Source: CAD feature listing. Evaluate the final solid. Frame: model axes, mm. Face numbers are marked on the shaded views. A direction names the side the tool comes from. Give positions to 0.01 mm unless a question says otherwise; leave off trailing zeros. Order: outer loops, then holes, each group sorted by start corner. A loop starts at its lowest first (then second) coordinate and runs counter-clockwise, first axis right, second up. Notation, with made-up numbers: (-38, -22) -> (17, -22) arc R23 cw to (17, 5) -> close; hole circle Ø6 at (34, 24). An arc over 180 degrees is marked (long way). Use CSV: the item, a comma, the result in double quotes.
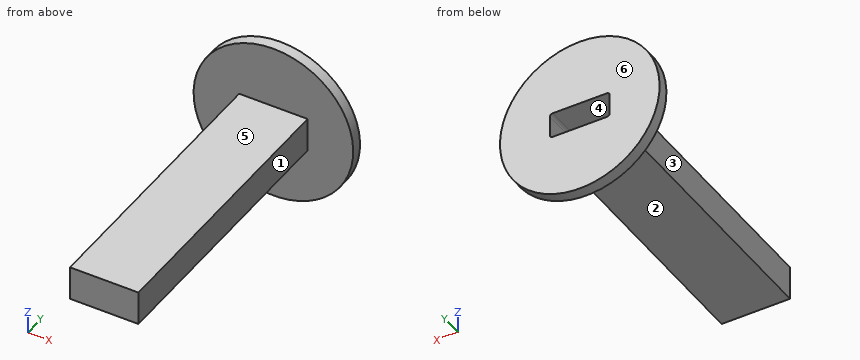
```python
from build123d import *

# Parameters (mm, degrees)
SKETCH1_R           = 88.9
BOSS_EXTRUDE1_DEPTH = 12.7
SKETCH2_W           = 76.2
SKETCH2_H           = 38.1
BOSS_EXTRUDE2_DEPTH = 314.325
CUT_EXTRUDE1_DEPTH  = 317.5


with BuildPart() as part:
    # Sketch1 → Boss-Extrude1 (new body)
    with BuildSketch(Plane(origin=(0, 0, 0), x_dir=(1, 0, 0), z_dir=(0, 1, 0))):
        with Locations(Location((0, 0, 0), (0, 0, 270))):
            Circle(SKETCH1_R)
    extrude(amount=BOSS_EXTRUDE1_DEPTH)

    # Sketch2 → Boss-Extrude2 (add)
    with BuildSketch(Plane.XZ):
        Rectangle(SKETCH2_W, SKETCH2_H)
    extrude(amount=BOSS_EXTRUDE2_DEPTH)

    # Sketch3 → Cut-Extrude1 (cut)
    with BuildSketch(Plane(origin=(0, 12.7, 0), x_dir=(1, 0, 0), z_dir=(0, 1, 0))):
        with BuildLine():
            Line((-30.1625, 14.2875), (30.1625, 14.2875))
            ThreePointArc((30.1625, 14.2875), (32.40756403, 13.35756403), (33.3375, 11.1125))
            Line((33.3375, 11.1125), (33.3375, -11.1125))
            ThreePointArc((33.3375, -11.1125), (32.40756403, -13.35756403), (30.1625, -14.2875))
            Line((30.1625, -14.2875), (-30.1625, -14.2875))
            ThreePointArc((-30.1625, -14.2875), (-32.40756403, -13.35756403), (-33.3375, -11.1125))
            Line((-33.3375, -11.1125), (-33.3375, 11.1125))
            ThreePointArc((-33.3375, 11.1125), (-32.40756403, 13.35756403), (-30.1625, 14.2875))
        make_face()
    extrude(amount=-CUT_EXTRUDE1_DEPTH, mode=Mode.SUBTRACT)


solid = part.part
```
1. Mould query, pull axis Z, two halves, no side actions, for the marked faces 4, 5 and 6. Classes: released by +Z, released by -Z, zero draft, split by the parting line, or undercut.
Answer below:
face 4,"undercut"
face 5,"released by +Z"
face 6,"zero draft"
2. Pin query (flat end, axial travel): P1, Ø6.5, axis at y = -98, z = 5, coming from the -X side; P2, Ø3, axis at y = -146, z = -22, coming from the -X side; P3, Ø8.5, axis at x = -3, z = 6, coming from the +Y side; P4, Ø23, axis at x = 1, y = -194.5, coming from the -Z side. Return the tip coordinate at first contact, or that it passes through.
Answer below:
P1,"stops at x = -38.1"
P2,"passes through"
P3,"stops at y = -304.8"
P4,"stops at z = -19.05"
3. Access query for the marked faces 1, 2 and 3. Directions: +Z, -Z, +X, -X, +Y, -Y. A direction counts if a zero-diameter tool reaches every point of the face in a straight line with its end or side. Return the directions, or none.
Answer below:
face 1,"+Z, -Z, +X, -Y"
face 2,"-Z, +X, -X, -Y"
face 3,"+Z, -Z, -X, -Y"
4. Section query B-B on z = 0. Return loops of the section in (x, y) (1 decimal), plus the area to 3 significant figures.
Answer below:
outline,"(-88.9, 0) -> (-38.1, 0) -> (-38.1, -314.3) -> (38.1, -314.3) -> (38.1, 0) -> (88.9, 0) -> (88.9, 12.7) -> (33.3, 12.7) -> (33.3, -304.8) -> (-33.3, -304.8) -> (-33.3, 12.7) -> (-88.9, 12.7) -> close"
area,"5,040 mm²"
5. Ray query, line 1 along Z through (x, y) = (6.5, -201); line 2 along X through (y, z) = (-21.5, 5.5); line 3 along Z through (x, y) = (-36, -272). Return the intervals inside material, ascending.
Answer below:
line 1,"z = -19.05 to -14.29, 14.29 to 19.05"
line 2,"x = -38.1 to -33.34, 33.34 to 38.1"
line 3,"z = -19.05 to 19.05"
6. Section query D-D on x = -73. Return loops of the section in (y, z).
Answer below:
outline,"(0, -50.74) -> (12.7, -50.74) -> (12.7, 50.74) -> (0, 50.74) -> close"
